Geometry: final body of the model. Coordinates: model frame, mm. Give positions to 0.01 mm unless a question says otherwise; leave off trailing zeros. Write each loop counter-clockwise with the first axis right and the second up, starting at its lowest first coordinate (ties: lowest second). Pieces come first, ordered by that corner, then holes.
Q1. Cut plane A-A on y = 229.5. Return the cut outline in (x, z).
Q2. Pin query (flat end, axial travel): pin 1 (3 mm diameter, centred on x = 0, y = 103, fed in from +Z). Return the tip coordinate at first contact, or that it passes through.
Q3. Line query: L1, parallel to Z at x = -3, y = 250; L2, parallel to Z at x = 7.25, y = 134. Output: solid intervals per line, ascending.
```python
from build123d import *

# Parameters (mm, degrees)
SKETCH_1_W          = 15
SKETCH_1_H          = 15
SKETCH_1_W_2        = 13
SKETCH_1_H_2        = 13
EXTRUDE_1_DEPTH     = 465
SKETCH_2_R          = 1.95
SKETCH_2_R_2        = 1.45
CUT_EXTRUDE_1_DEPTH = 466.302321077
SKETCH_3_R          = 1.45
CUT_EXTRUDE_2_DEPTH = 466.302321077


with BuildPart() as part:
    # 草图1 → 拉伸-薄壁1 (new body)
    with BuildSketch(Plane(origin=(0, 0, 0), x_dir=(1, 0, 0), z_dir=(0, 1, 0))):
        Rectangle(SKETCH_1_W, SKETCH_1_H)
        Rectangle(SKETCH_1_W_2, SKETCH_1_H_2, mode=Mode.SUBTRACT)
    extrude(amount=EXTRUDE_1_DEPTH)

    # 草图2 → 切除-拉伸1 (cut, through all)
    with BuildSketch(Plane.XY.offset(7.5)):
        with Locations((0, 118)):
            Circle(SKETCH_2_R)
        with Locations((0, 103)):
            Circle(SKETCH_2_R)
        with Locations((0, 134)):
            Circle(SKETCH_2_R_2)
        with Locations((0, 127)):
            Circle(SKETCH_2_R_2)
        with Locations((0, 322.5)):
            Circle(SKETCH_2_R_2)
        with Locations((0, 315.5)):
            Circle(SKETCH_2_R_2)
    extrude(amount=-CUT_EXTRUDE_1_DEPTH, mode=Mode.SUBTRACT)

    # 草图3 → 切除-拉伸2 (cut, through all)
    with BuildSketch(Plane(origin=(7.5, 0, 0), x_dir=(0, 0, -1), z_dir=(1, 0, 0))):
        with Locations((0, 457.5)):
            Circle(SKETCH_3_R)
        with Locations((0, 437.5)):
            Circle(SKETCH_3_R)
        with Locations((0, 134)):
            Circle(SKETCH_3_R)
        with Locations((0, 127)):
            Circle(SKETCH_3_R)
        with Locations((0, 315.5)):
            Circle(SKETCH_3_R)
        with Locations((0, 322.5)):
            Circle(SKETCH_3_R)
        with Locations((0, 7.5)):
            Circle(SKETCH_3_R)
        with Locations((0, 27.5)):
            Circle(SKETCH_3_R)
    extrude(amount=-CUT_EXTRUDE_2_DEPTH, mode=Mode.SUBTRACT)


solid = part.part
```
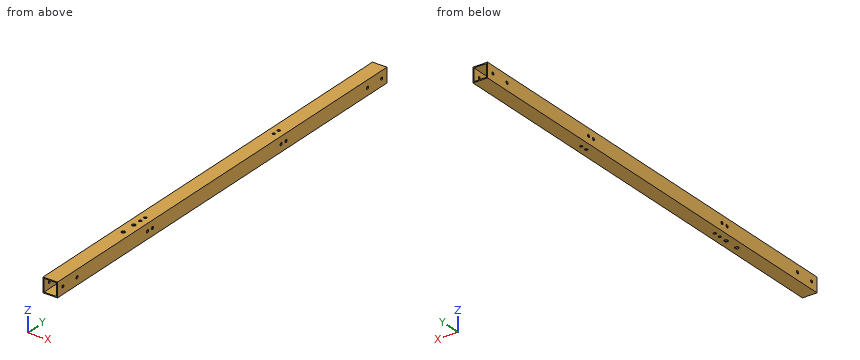
Data:
1. outline: (-7.5, -7.5) - (7.5, -7.5) - (7.5, 7.5) - (-7.5, 7.5) - close; hole (-6.5, -6.5) - (6.5, -6.5) - (6.5, 6.5) - (-6.5, 6.5) - close
2. pin 1: passes through
3. L1: z = -7.5 to -6.5, 6.5 to 7.5
3. L2: z = -7.5 to -1.45, 1.45 to 7.5
